from build123d import *

# Parameters (mm, degrees)
SKETCH1_W           = 38.65
SKETCH1_H           = 23
BOSS_EXTRUDE1_DEPTH = 31.5
CUT_EXTRUDE1_DEPTH  = 20
SKETCH4_R           = 0.8
CUT_EXTRUDE2_DEPTH  = 2.15
BOSS_EXTRUDE2_START = -6
SKETCH6_W           = 37.65
SKETCH6_H           = 8
SKETCH6_R           = 1.5
SKETCH6_W_2         = 1
BOSS_EXTRUDE2_DEPTH = 7.5


with BuildPart() as part:
    # Sketch1 → Boss-Extrude1 (new body)
    with BuildSketch(Plane(origin=(0, 0, 0), x_dir=(1, 0, 0), z_dir=(0, 1, 0))):
        with Locations((19.325, 11.5)):
            Rectangle(SKETCH1_W, SKETCH1_H)
    extrude(amount=BOSS_EXTRUDE1_DEPTH)

    # Sketch3 → Cut-Extrude1 (cut)
    with BuildSketch(Plane.XY):
        Polygon((2, 25.5), (2, 6), (4, 6), (4, 3), (36.5, 3), (36.5, 8.2), (37.65, 8.2), (37.65, 23.3), (36.5, 23.3), (36.5, 28.5), (4, 28.5), (4, 25.5), align=None)
    extrude(amount=-CUT_EXTRUDE1_DEPTH, mode=Mode.SUBTRACT)

    # Sketch4 → Cut-Extrude2 (cut)
    with BuildSketch(Plane.ZY.offset(-36.5)):
        with Locations((-14, 26.55)):
            Circle(SKETCH4_R)
        with Locations((-14, 6.05)):
            Circle(SKETCH4_R)
    extrude(amount=-CUT_EXTRUDE2_DEPTH, mode=Mode.SUBTRACT)

    # Sketch6 → Boss-Extrude2 (add)
    # profile 1 of 2: a face of its own
    with BuildSketch(Plane.XZ.offset(BOSS_EXTRUDE2_START)):
        with Locations((18.825, -27)):
            Rectangle(SKETCH6_W, SKETCH6_H)
        with Locations(Location((8, -27, 0), (0, 0, 270))):
            Circle(SKETCH6_R, mode=Mode.SUBTRACT)
        with Locations(Location((29.65, -27, 0), (0, 0, 270))):
            Circle(SKETCH6_R, mode=Mode.SUBTRACT)
    # profile 2 of 2: a face of its own
    with BuildSketch(Plane.XZ.offset(BOSS_EXTRUDE2_START)):
        with Locations((38.15, -27)):
            Rectangle(SKETCH6_W_2, SKETCH6_H)
    extrude(amount=-BOSS_EXTRUDE2_DEPTH)


solid = part.part
Geometry check sheet. Reference: the model listing, model coordinates, mm. A direction names the side the tool comes from. Round coordinates to 2 decimals unless told otherwise and drop trailing zeros. Write each loop counter-clockwise with the first axis right and the second up, starting at its lowest first coordinate (ties: lowest second). Pieces come first, ordered by that corner, then holes. Notation, with made-up numbers: (16, 61) -> (34, 61) arc R16 cw to (34, 69) -> close; hole circle Ø7 at (-39, 12.5). An arc over 180 degrees is marked (long way). One line per item, written item: value. Start each with the question number.
(1) Draft check along X on faces 1 (the flat face through (19, 3, -23)), 2 (the flat face through (20, 28.5, -10)). Enter one of: +X half, -X half, draft (parallel to the pull), parting line (faces both ways), or undercut.
(2) Cross-section at C-C, the plane x = 8. Record the cut outline in (y, z).
(3) Cross-section at D-D, the plane z = -14. Record the cut outline in (x, y).
(4) Go/stop test with flat-tipped pins: pin 1 Ø4 at (x, z) = (8, -27) entering from -Y; pin 2 Ø5 at (x, z) = (29.65, -27) entering from +Y. Record where each tip stops, or that it passes through.
(5) Cross-section at B-B, the plane y = 26.55. Record the cut outline in (x, z).
(6) Cross-section at A-A, the plane z = -27. Record the cut outline in (x, y), and give its area (3 significant figures).
(7) Scan lines: line 1 (X direction, y = 8, z = -27); line 2 (Y direction, x = 37.75, z = -14); line 3 (X direction, y = 7, z = -10.5). Record each from-to range of solid material in increasing order. Write a range as [from, to].
(8) Access from +Z, -Z, +X, -X, +Y, -Y to the whole of each face (thin tool, end or side, straight path). Record for faces 3 (the flat face through (19, 6, -27)), 4 (the flat face through (37, 8.2, -10)), 5 (the flat face through (19, 13.5, -27)), 6 (the cylindrical face through (28.74, 9.7, -25.81)).
Answer:
1. face 1: draft
1. face 2: undercut
2. outline: (0, -23) -> (6, -23) -> (6, -25.5) -> (13.5, -25.5) -> (13.5, -23) -> (31.5, -23) -> (31.5, 0) -> (28.5, 0) -> (28.5, -20) -> (3, -20) -> (3, 0) -> (0, 0) -> close; (6, -31) -> (13.5, -31) -> (13.5, -28.5) -> (6, -28.5) -> close
3. outline: (0, 0) -> (38.65, 0) -> (38.65, 5.25) -> (36.5, 5.25) -> (36.5, 3) -> (4, 3) -> (4, 6) -> (2, 6) -> (2, 25.5) -> (4, 25.5) -> (4, 28.5) -> (36.5, 28.5) -> (36.5, 27.35) -> (38.65, 27.35) -> (38.65, 31.5) -> (0, 31.5) -> close; (36.5, 6.85) -> (38.65, 6.85) -> (38.65, 25.75) -> (36.5, 25.75) -> (36.5, 23.3) -> (37.65, 23.3) -> (37.65, 8.2) -> (36.5, 8.2) -> close
4. pin 1: y = 6
4. pin 2: y = 13.5
5. outline: (0, -23) -> (38.65, -23) -> (38.65, -14.8) -> (36.5, -14.8) -> (36.5, -20) -> (4, -20) -> (4, 0) -> (0, 0) -> close; (36.5, -13.2) -> (38.65, -13.2) -> (38.65, 0) -> (36.5, 0) -> close
6. outline: (0, 6) -> (6.5, 6) -> (6.5, 13.5) -> (0, 13.5) -> close; (9.5, 6) -> (28.15, 6) -> (28.15, 13.5) -> (9.5, 13.5) -> close; (31.15, 6) -> (38.65, 6) -> (38.65, 13.5) -> (31.15, 13.5) -> close
6. area: 245 mm²
7. line 1: [0, 6.5], [9.5, 28.15], [31.15, 38.65]
7. line 2: [0, 5.25], [6.85, 25.75], [27.35, 31.5]
7. line 3: [0, 2], [36.5, 38.65]
8. face 3: -Z, +X, -X, -Y
8. face 4: +Z
8. face 5: -Z, +X, -X, +Y
8. face 6: +Y, -Y
